For this review, use the dimensioned drawing (mm, ordinates from the lowest corner) and the shaded views. A direction names the side the tool comes from. Round coordinates to 2 decimals unless told otherwise and drop trailing zeros. Write each loop counter-clockwise with the first axis right and the second up, starting at its lowest first coordinate (ties: lowest second). Pieces come first, ordered by that corner, then holes. Notation, with made-up numbers: (-26.5, 71) - (0.5, 71) arc R15 cw to (0.5, 93) - close; hole circle Ø2 at (7.25, 85.25). An arc over 180 degrees is marked (long way). Return JSON: item names as keys, results as strings.
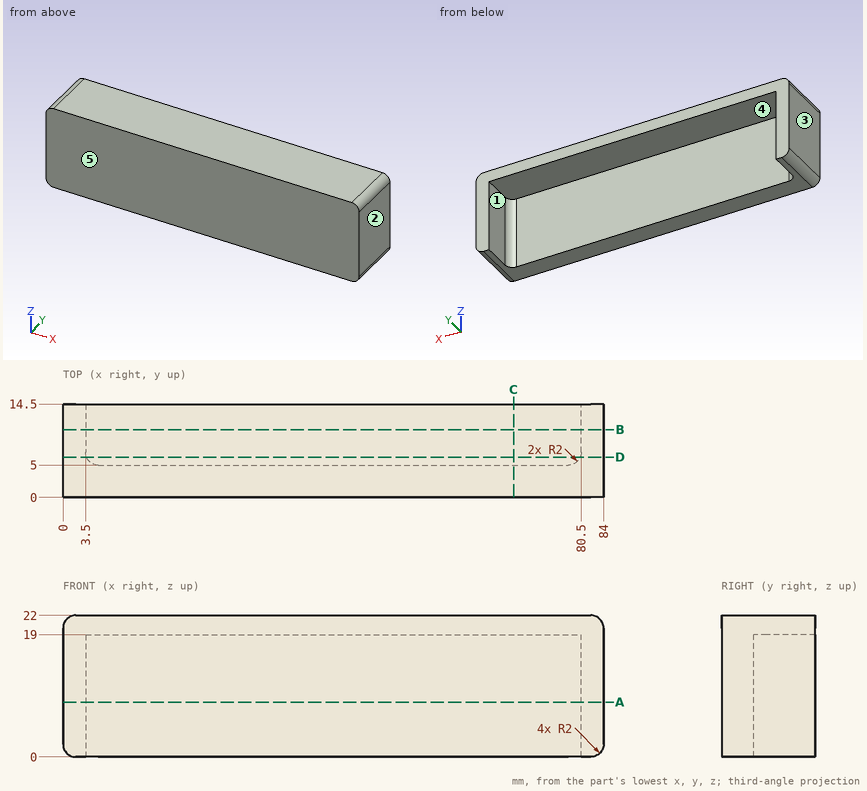
(1) Wall thickness on line 1 (X direction, y = 9.5, z = 3.75); line 2 (Y direction, x = 33, z = 10); line 3 (Z direction, x = 40, y = 7.25): over which ranges is each line inside the solid? List them lowest first.
Filled in:
{"line 1": "x = 0 to 3.5, 80.5 to 84", "line 2": "y = 0 to 5", "line 3": "z = 19 to 22"}
(2) Add section B-B (y = 10.5). Write out the cut boundary in (x, z).
Filled in:
{"outline": "(0, 2) arc R2 ccw to (2, 0) - (3.5, 0) - (3.5, 19) - (80.5, 19) - (80.5, 0) - (82, 0) arc R2 ccw to (84, 2) - (84, 20) arc R2 ccw to (82, 22) - (2, 22) arc R2 ccw to (0, 20) - close"}
(3) Clearance check with flat-ended pins moving along their axes: pin 1 Ø4 at (x, y) = (46, 7.5) entering from -Z; pin 2 Ø4 at (x, z) = (55.5, 10) entering from +Y; pin 3 Ø6 at (y, z) = (9.5, 14) entering from -X. State where each tip first meets the part, or that it passes through.
Filled in:
{"pin 1": "stops at z = 19", "pin 2": "stops at y = 5", "pin 3": "stops at x = 0"}
(4) Add section C-C (x = 70). Write out the cut boundary in (y, z), plus the area to 4 significant figures.
Filled in:
{"outline": "(0, 0) - (5, 0) - (5, 19) - (14.5, 19) - (14.5, 22) - (0, 22) - close", "area": "138.5 mm2"}
(5) Mouldability with a two-part tool opening along X and no side actions: class the marked faces 1, 2 and 3 as released by +X, released by -X, zero draft, split by the parting line, or undercut.
Filled in:
{"face 1": "undercut", "face 2": "released by +X", "face 3": "released by -X"}
(6) Add section D-D (y = 6.25). Write out the cut boundary in (x, z), plus the area to 3 significant figures.
Filled in:
{"outline": "(0, 2) arc R2 ccw to (2, 0) - (3.65, 0) - (3.65, 19) - (80.35, 19) - (80.35, 0) - (82, 0) arc R2 ccw to (84, 2) - (84, 20) arc R2 ccw to (82, 22) - (2, 22) arc R2 ccw to (0, 20) - close", "area": "387 mm2"}
(7) For the marked faces 4 and 5, list the 3-axis set-ups (+Z, -Z, +X, -X, +Y, -Y) from which the entire face can be reached by the end or side of a thin tool; tool diameter is ignored.
Filled in:
{"face 4": "-Z, +Y", "face 5": "+Z, -Z, +X, -X, -Y"}
(8) Add section A-A (z = 8.5). Write out the cut boundary in (x, y), plus the area to 3 significant figures.
Filled in:
{"outline": "(0, 0) - (84, 0) - (84, 14.5) - (80.5, 14.5) - (80.5, 7) arc R2 cw to (78.5, 5) - (5.5, 5) arc R2 cw to (3.5, 7) - (3.5, 14.5) - (0, 14.5) - close", "area": "488 mm2"}
